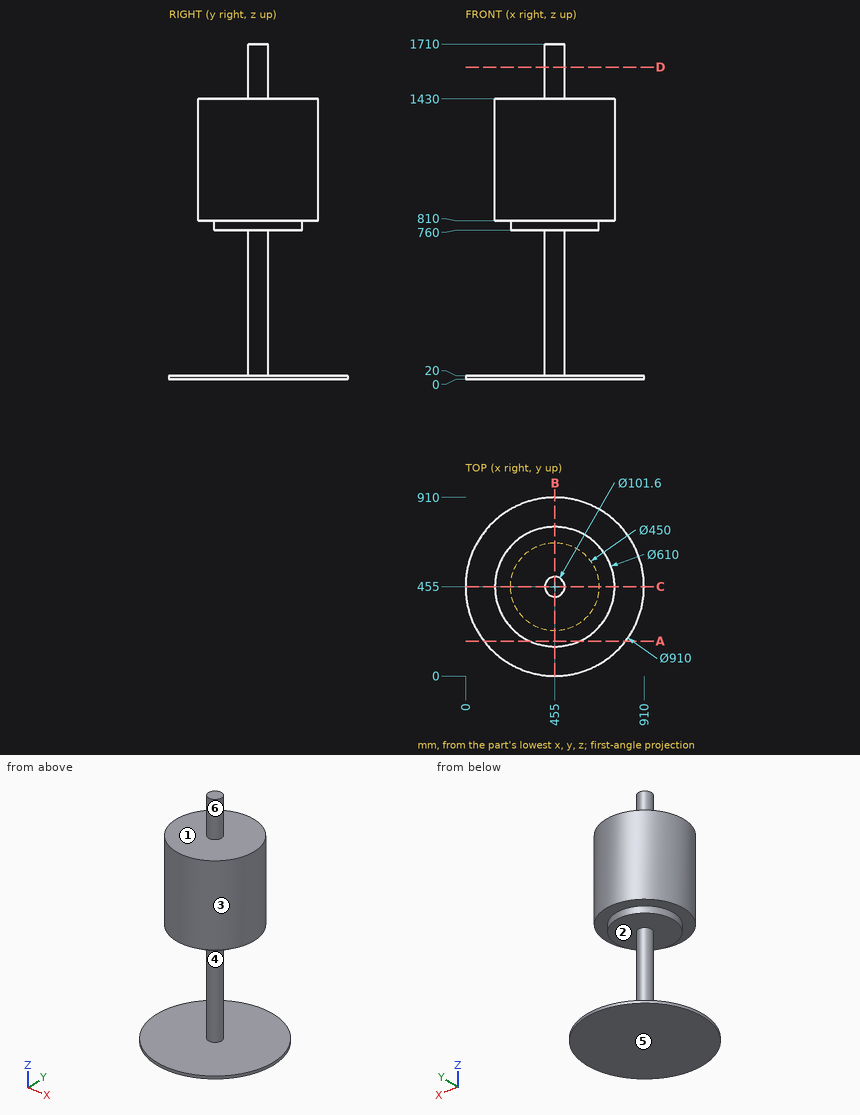
Could you check a few things on this drawing? It's one solid part, dimensions in mm from its lowest x, y, z. A direction names the side the tool comes from. Round coordinates to 2 decimals unless told otherwise and drop trailing zeros. Write each loop counter-clockwise with the first axis right and the second up, starting at its lowest first coordinate (ties: lowest second). Pieces come first, ordered by that corner, then holes. Notation, with made-up numbers: (64.25, -15) -> (119.25, -15) arc R35 cw to (119.25, 21) -> close; hole circle Ø8 at (49.25, -33). An arc over 180 degrees is marked (long way). Use a Markdown table: item, result.
1. If we section it at B-B (x = 455): List the corners of the cut face in (y, z) for me.
Answer key:
| item | result |
|---|---|
| outline | (0, 0) -> (910, 0) -> (910, 20) -> (505.8, 20) -> (505.8, 760) -> (680, 760) -> (680, 810) -> (760, 810) -> (760, 1430) -> (505.8, 1430) -> (505.8, 1710) -> (404.2, 1710) -> (404.2, 1430) -> (150, 1430) -> (150, 810) -> (230, 810) -> (230, 760) -> (404.2, 760) -> (404.2, 20) -> (0, 20) -> close |
2. We'd pull the mould along Z, two halves only. Please class the marked faces 1, 2 and 3: +Z half, -Z half, draft (parallel to the pull), parting line (faces both ways), or undercut.
Answer key:
| item | result |
|---|---|
| face 1 | +Z half |
| face 2 | undercut |
| face 3 | draft |
3. If we section it at A-A (y = 178): List the corners of the cut face in (x, z) for me.
Answer key:
| item | result |
|---|---|
| outline | (94.03, 0) -> (815.97, 0) -> (815.97, 20) -> (94.03, 20) -> close; (327.34, 810) -> (582.66, 810) -> (582.66, 1430) -> (327.34, 1430) -> close |
4. Which directions (+Z, -Z, +X, -X, +Y, -Y) give clear straight access to the entire face, cutting with the end or side of a thin tool? Please do the marked faces 4, 5 and 6.
Answer key:
| item | result |
|---|---|
| face 4 | none |
| face 5 | -Z, +X, -X, +Y, -Y |
| face 6 | +Z |
5. If we section it at D-D (z = 1592.5): List the corners of the cut face in (x, y) for me, then the cut area to 3 significant figures.
Answer key:
| item | result |
|---|---|
| outline | circle Ø101.6 at (455, 455) |
| area | 8,110 mm^2 |
6. Please list where these lines run through material, in increasing order: probe 1 along Z at (x, y) = (713, 406); probe 2 along Z at (x, y) = (547, 419.5); probe 3 along Y at (x, z) = (440, 1056.5).
Answer key:
| item | result |
|---|---|
| probe 1 | z = 0 to 20, 810 to 1430 |
| probe 2 | z = 0 to 20, 760 to 1430 |
| probe 3 | y = 150.37 to 759.63 |
7. For pin 1 Ø4 at (x, z) = (203.5, 1028) entering from -Y; pin 2 Ø4 at (x, y) = (227.5, 220) entering from +Z; pin 3 Ø10 at (y, z) = (211, 1094.5) entering from -X, each with a flat end and sliding along its axis, tell me the tip position at first contact or that it passes through.
Answer key:
| item | result |
|---|---|
| pin 1 | stops at y = 279.57 |
| pin 2 | stops at z = 20 |
| pin 3 | stops at x = 265.52 |
